Geometry check sheet. Reference: the model listing, model coordinates, mm. Face numbers are marked on the shaded views. A direction names the side the tool comes from. Round coordinates to 2 decimals unless told otherwise and drop trailing zeros. Write each loop counter-clockwise with the first axis right and the second up, starting at its lowest first coordinate (ties: lowest second). Pieces come first, ordered by that corner, then holes. Notation, with made-up numbers: (48.25, -36) -> (85.25, -36) arc R14 ccw to (85.25, -25) -> close; hole circle Ø7 at (38.25, -22). An arc over 180 degrees is marked (long way). Put each result on its own line as item: value. Start each with the question number.
from build123d import *

# Parameters (mm, degrees)
SKETCH1_R                = 1.125
SKETCH1_R_2              = 7.05
BOSS_EXTRUDE1_DEPTH      = 5
BOSS_EXTRUDE2_DEPTH      = 8
BOSS_EXTRUDE2_DEPTH_BACK = 30
SKETCH2_W                = 26
SKETCH2_H                = 4
FILLET1_R                = 4
FILLET2_R                = 4
CUT_EXTRUDE1_DEPTH       = 44.703546767
CUT_EXTRUDE1_DEPTH_BACK  = 44.703546767
SKETCH3_R                = 1
CUT_EXTRUDE3_OUTLINE_R   = 1
CUT_EXTRUDE3_DEPTH       = 4.0000001


with BuildPart() as part:
    # Sketch1 → Boss-Extrude1 (new body)
    with BuildSketch(Plane(origin=(0, 0, 0), x_dir=(0, 0, -1), z_dir=(1, 0, 0))):
        with BuildLine():
            Line((-13, 0), (-13, -20))
            Line((-13, -20), (13, -20))
            Line((13, -20), (13, 0))
            ThreePointArc((13, 0), (0, 13), (-13, 0))
        make_face()
        with Locations((0, 9)):
            Circle(SKETCH1_R, mode=Mode.SUBTRACT)
        with Locations((9, 0)):
            Circle(SKETCH1_R, mode=Mode.SUBTRACT)
        with Locations((0, -9)):
            Circle(SKETCH1_R, mode=Mode.SUBTRACT)
        with Locations((-9, 0)):
            Circle(SKETCH1_R, mode=Mode.SUBTRACT)
        Circle(SKETCH1_R_2, mode=Mode.SUBTRACT)
    extrude(amount=BOSS_EXTRUDE1_DEPTH)

    # Sketch2 → Boss-Extrude2 (add, two sides: drawn at the far end of the back side and taken through both)
    with BuildSketch(Plane.ZY.offset(-BOSS_EXTRUDE2_DEPTH_BACK)):
        with Locations((0, -18)):
            Rectangle(SKETCH2_W, SKETCH2_H)
    extrude(amount=BOSS_EXTRUDE2_DEPTH + BOSS_EXTRUDE2_DEPTH_BACK)

    # Fillet1
    fillet1_edges = [part.edges().sort_by_distance(p)[0] for p in [
        (5, -16, 0),
        (0, -16, 0),
    ]]
    fillet(fillet1_edges, radius=FILLET1_R)

    # Fillet2
    fillet2_edges = [part.edges().sort_by_distance(p)[0] for p in [
        (30, -18, -13),
        (30, -18, 13),
        (-8, -18, -13),
        (-8, -18, 13),
    ]]
    fillet(fillet2_edges, radius=FILLET2_R)

    # Sketch3 → Cut-Extrude1 (cut, two sides: drawn at the far end of the back side and taken through both)
    with BuildSketch(Plane(origin=(0, -16, 0), x_dir=(1, 0, 0), z_dir=(0, 1, 0)).offset(-CUT_EXTRUDE1_DEPTH_BACK)):
        with Locations(Location((-4, -9, 0), (0, 0, 270.000000003))):
            Circle(SKETCH3_R)
        with Locations(Location((-4, 9, 0), (0, 0, 270.000000003))):
            Circle(SKETCH3_R)
        with Locations(Location((26, 9, 0), (0, 0, 270))):
            Circle(SKETCH3_R)
        with Locations(Location((26, -9, 0), (0, 0, 270))):
            Circle(SKETCH3_R)
    extrude(amount=CUT_EXTRUDE1_DEPTH + CUT_EXTRUDE1_DEPTH_BACK, mode=Mode.SUBTRACT)

    # Cut-Extrude3: read off the stored shape, not the designer's step
    # Cut-Extrude3 outline → Cut-Extrude3 (cut)
    with BuildSketch(Plane(origin=(0, -16, 0), x_dir=(1, 0, 0), z_dir=(0, 1, 0))):
        with BuildLine():
            Line((-4, -6.5), (-4, 6.5))
            ThreePointArc((-4, 6.5), (-1.5, 9), (-4, 11.5))
            Line((-4, 11.5), (-4, 13))
            ThreePointArc((-4, 13), (-6.828427125, 11.828427125), (-8, 9))
            Line((-8, 9), (-8, -9))
            ThreePointArc((-8, -9), (-6.828427125, -11.828427125), (-4, -13))
            Line((-4, -13), (-4, -11.5))
            ThreePointArc((-4, -11.5), (-1.5, -9), (-4, -6.5))
        make_face()
        with Locations((-4, -9)):
            Circle(CUT_EXTRUDE3_OUTLINE_R, mode=Mode.SUBTRACT)
        with Locations((-4, 9)):
            Circle(CUT_EXTRUDE3_OUTLINE_R, mode=Mode.SUBTRACT)
    extrude(amount=CUT_EXTRUDE3_DEPTH, mode=Mode.SUBTRACT)


solid = part.part
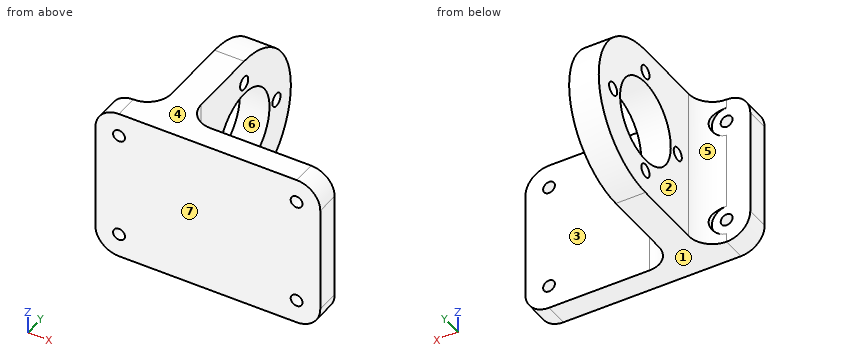
(1) Set-up check for the marked faces 1, 2 and 3: record each of +Z, -Z, +X, -X, +Y, -Y from which the full face is reachable in a straight line by a thin tool's end or side.
(2) Go/stop test with flat-tipped pins: pin 1 Ø8 at (y, z) = (-10, -2) entering from +X; pin 2 Ø8 at (y, z) = (-8, -7) entering from -X; pin 3 Ø7.5 at (y, z) = (1, 6) entering from +X; pin 4 Ø1.2 at (x, z) = (-4, 9) entering from -Y. Record where each tip stops, or that it passes through.
(3) Sectioned sample at C-C (z = 0). Record the cut outline in (x, y) (3 decimals).
(4) Mould release check, pull along Y, two halves, no side actions. Record for the marked faces 4, 5, 6 and 7: +Y half, -Y half, draft (parallel to the pull), parting line (faces both ways), or undercut.
(5) Sectioned sample at D-D (y = 9). Record the cut outline in (x, z) (3 decimals), and give its area (3 significant figures).
(6) Material ranges on L1, parallel to Y at x = 3.7, z = 0 (3 decimals); L2, parallel to X at y = -18.2, z = 9; L3, parallel to Y at x = 15, z = 6.25, recorded low to high. Write a range as from..to.
(7) Sectioned sample at A-A (y = -9). Record the cut outline in (x, z) (3 decimals).
(8) Sectioned sample at B-B (x = 3). Record the cut outline in (y, z) (3 decimals), and give its area (3 significant figures).
Found:
1. face 1: -Z, +X, -X, +Y, -Y
1. face 2: +Z, -Z, -X, +Y
1. face 3: +Z, -Z, +X, +Y
2. pin 1: x = 5.54
2. pin 2: x = 0
2. pin 3: x = 5
2. pin 4: through
3. outline: (-8, -20) -> (30, -20) -> (30, -16) -> (9, -16) arc R4 cw to (5, -12) -> (5, -10.125) -> (0, -10.125) -> (0, -12) arc R4 cw to (-4, -16) -> (-8, -16) -> close; (0, -7.875) -> (5, -7.875) -> (5, -7.05) -> (0, -7.05) -> close; (0, 7.05) -> (5, 7.05) -> (5, 7.875) -> (0, 7.875) -> close; (0, 10.125) -> (5, 10.125) -> (5, 13) -> (0, 13) -> close
4. face 4: draft
4. face 5: +Y half
4. face 6: undercut
4. face 7: -Y half
5. outline: (0, -9.381) -> (5, -9.381) -> (5, -1.125) -> (0, -1.125) -> close; (0, 1.125) -> (5, 1.125) -> (5, 9.381) -> (0, 9.381) -> close
5. area: 82.6 mm2
6. L1: -20..-10.125, -7.875..-7.05, 7.05..7.875, 10.125..13
6. L2: -8..-5, -3..25, 27..30
6. L3: -20..-16
7. outline: (0, -13) -> (5, -13) -> (5, -1.125) -> (0, -1.125) -> close; (0, 1.125) -> (5, 1.125) -> (5, 13) -> (0, 13) -> close
8. outline: (-20, -13) -> (0, -13) arc R13 ccw to (0, 13) -> (-20, 13) -> close; hole circle Ø2.25 at (-9, 0); hole circle Ø14.1 at (0, 0); hole circle Ø2.25 at (0, -9); hole circle Ø2.25 at (0, 9); hole circle Ø2.25 at (9, 0)
8. area: 613 mm2
